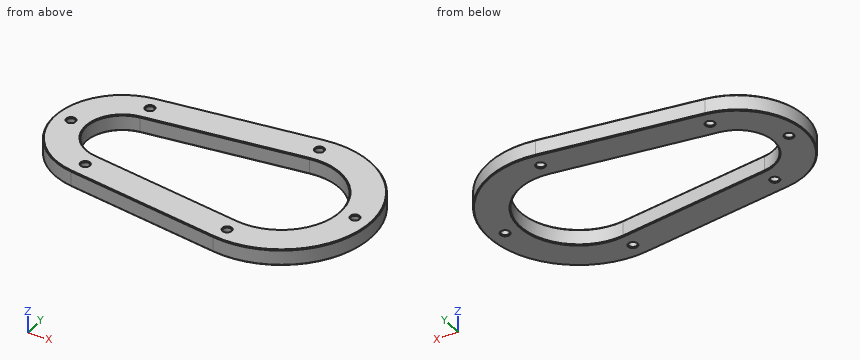
Autodesk Inventor part; units mm, degrees
ref_plane "YZ Plane" through (0, 0, 0) normal (1, 0, 0) x (0, 1, 0)
ref_plane "XZ Plane" through (0, 0, 0) normal (0, 1, 0) x (-1, 0, 0)
ref_plane "XY Plane" through (0, 0, 0) normal (0, 0, 1) x (1, 0, 0)
sketch "Sketch1" plane through (0, 0, 0) normal (0, 0, 1) x (1, 0, 0)
  arc A0 (-5.9149, 42.0864) -> (-5.9149, -42.0864) centre (0, 0) ccw
  arc A1 (92.2885, -55.888) -> (92.2885, 55.888) centre (100.143, 0) ccw
  line L0 (-42.5, 0) -> (156.5802, 0)
  line L1 (92.2885, 55.888) -> (-5.9149, 42.0864)
  line L2 (-5.9149, -42.0864) -> (92.2885, -55.888)
  line L3 (-3.1314, 22.281) -> (95.0719, 36.0826)
  arc A2 (95.0719, -36.0826) -> (95.0719, 36.0826) centre (100.143, 0) ccw
  line L4 (95.0719, -36.0826) -> (-3.1314, -22.281)
  arc A3 (-3.1314, 22.281) -> (-3.1314, -22.281) centre (0, 0) ccw
  point P0 (146.5802, 0)
  point P1 (95.0719, 46.1809)
  point P2 (95.0719, -46.1809)
  point P3 (-32.5, 0)
  point P4 (-3.1314, 32.3793)
  point P5 (-3.1314, -32.3793)
  dimension "d0" = 85
  dimension "d1" = 100.143
  dimension "d2" = 8
  dimension "d3" = 20
  dimension "d4" = 10
  dimension "d5" = 10
  dimension "d6" = 10
  dimension "d7" = 10
  dimension "d8" = 10
  dimension "d9" = 10
extrude "Extrusion1" add sketch "Sketch1" along normal blind 10 contours L1 A1 L0 A2 L3 A3 A0 | L0 A3 L4 A2 A1 L2 A0
hole "Hole1" at (-32.5, 0, 0) at (-3.1314, 32.3793, 0) at (95.0719, 46.1809, 0) at (146.5802, 0, 0) at (95.0719, -46.1809, 0) at (-3.1314, -32.3793, 0) direction (0, 0, 1) diameter 5 end through all
chamfer "Chamfer1" distance 0.5 angle 45 28 edges at (136.5802, 0, 10) (45.9703, -29.1818, 10) (-22.5, 0, 10) (45.9703, 29.1818, 10) (136.5802, 0, 0) (45.9703, -29.1818, 0) (-22.5, 0, 0) (45.9703, 29.1818, 0) (-3.1314, -34.8793, 0) (-32.5, -2.5, 0) (95.0719, -48.6809, 0) (146.5802, -2.5, 0) (-3.1314, 29.8793, 0) (95.0719, 43.6809, 0) (-3.1314, -34.8793, 10) (-32.5, -2.5, 10) (95.0719, -48.6809, 10) (146.5802, -2.5, 10) (-3.1314, 29.8793, 10) (95.0719, 43.6809, 10) (156.5802, 0, 0) (43.1868, 48.9872, 0) (-42.5, 0, 0) (43.1868, -48.9872, 0) (156.5802, 0, 10) (43.1868, 48.9872, 10) (-42.5, 0, 10) (43.1868, -48.9872, 10)
properties part number "spacerBase" material "Aluminum 6061"
Could you check a few things on this model? Use its own coordinates, in mm. Give positions to 0.01 mm unless a question says otherwise; leave off trailing zeros. Order: outer loops, then holes, each group sorted by start corner. A loop starts at its lowest first (then second) coordinate and runs counter-clockwise, first axis right, second up.
Q1. Suppose I cut it at C-C, the plane z = 3. Write out the boundary of the cut face in (x, y).
Q2. Suppose I cut it at A-A, the plane y = 0. Count the separate pieces of the cut face and the enclosed holes in it, and give its area (3 significant figures).
Q3. If I drill on line 1 along X through (y, z) = (0, 4.5); line 2 along Y through (x, z) = (-4, 7.5); line 3 along Y through (x, z) = (23.5, 5), over which ranges is the centre line in solid material (lowest first)?
Q4. Suppose I cut it at B-B, the plane x = 2.5. Write out the boundary of the cut face in (y, z).
Q5. I'm going to push flat-ended pins straight in: P1, Ø1, axis at x = 15, z = 2, coming from the +Y side; P2, Ø4, axis at y = 4.5, z = 3.5, coming from the -X side; P3, Ø3, axis at x = 95.07, y = 46.18, coming from the -Z side; P4, Ø3, axis at y = -45, z = 4.5, coming from the +X side. Where does each tip first touch, or does it pass through?
Solution:
1. outline: (-5.91, -42.09) - (92.29, -55.89) arc R56.44 ccw (long way) to (92.29, 55.89) - (-5.91, 42.09) arc R42.5 ccw to start; hole circle Ø5 at (-32.5, 0); hole circle Ø5 at (-3.13, -32.38); hole circle Ø5 at (-3.13, 32.38); hole (-3.13, -22.28) - (95.07, -36.08) arc R36.44 ccw (long way) to (95.07, 36.08) - (-3.13, 22.28) arc R22.5 ccw to start; hole circle Ø5 at (95.07, -46.18); hole circle Ø5 at (95.07, 46.18); hole circle Ø5 at (146.58, 0)
2. separate pieces: 4
2. enclosed holes: 0
2. area: 298 mm2
3. line 1: x = -42.5 to -35, -30 to -22.5, 136.58 to 144.08, 149.08 to 156.58
3. line 2: y = -42.36 to -34.72, -30.04 to -22.14, 22.14 to 30.04, 34.72 to 42.36
3. line 3: y = -46.22 to -26.02, 26.02 to 46.22
4. outline: (-43.27, 0.5) - (-42.76, 0) - (-23.58, 0) - (-23.07, 0.5) - (-23.07, 9.5) - (-23.58, 10) - (-42.76, 10) - (-43.27, 9.5) - close; (23.07, 0.5) - (23.58, 0) - (42.76, 0) - (43.27, 0.5) - (43.27, 9.5) - (42.76, 10) - (23.58, 10) - (23.07, 9.5) - close
5. P1: stops at y = 45.1
5. P2: stops at x = -42.43
5. P3: passes through
5. P4: stops at x = 136.1
